Input: dimensioned drawing with shaded views. Units: mm. Origin: part minimum x, y, z. A direction names the side the tool comes from. Give positions to 0.01 mm unless a question says otherwise; leave off trailing zeros. Order: outer loops, then holes, each group sorted by start corner. A loop starts at its lowest first (then second) coordinate and runs counter-clockwise, first axis right, second up. Notation, with made-up numbers: M -14.5,26.5 L 28.5,26.5 A26 cw 28.5,49.5 Z; hole C 11.25,8.25 d6. An arc over 180 degrees is marked long. Answer in a Markdown table with one row per item. Add a question column.
(1) Pin query (flat end, axial travel): P1, Ø3.5, axis at x = 6.35, z = 6.35, coming from the +Y side. Return the tip coordinate at first contact, or that it passes through.
(2) Mould query, pull axis Z, two halves, no side actions, for the marked faces 1, 2 and 3. Classes: pulls with the +Z half, pulls with the -Z half, needs draft (parallel to the pull), parting line crosses it, or undercut.
(3) Material intervals for line 1 along X through (y, z) = (3.5, 6.35); line 2 along Y through (x, z) = (3.25, 2); line 3 along X through (y, z) = (8.75, 6.75) (1 decimal), sorted ascending.
(4) Section query B-B, the plane x = 7. Return loops of the section in (y, z).
(5) Set-up query: the marked faces 4 and 5. Return all of +Z, -Z, +X, -X, +Y, -Y with unobstructed straight access to the full face (end or side cutting, diameter ignored); none if empty.
(6) Section query A-A, the plane z = 6.35. Return loops of the section in (x, y).
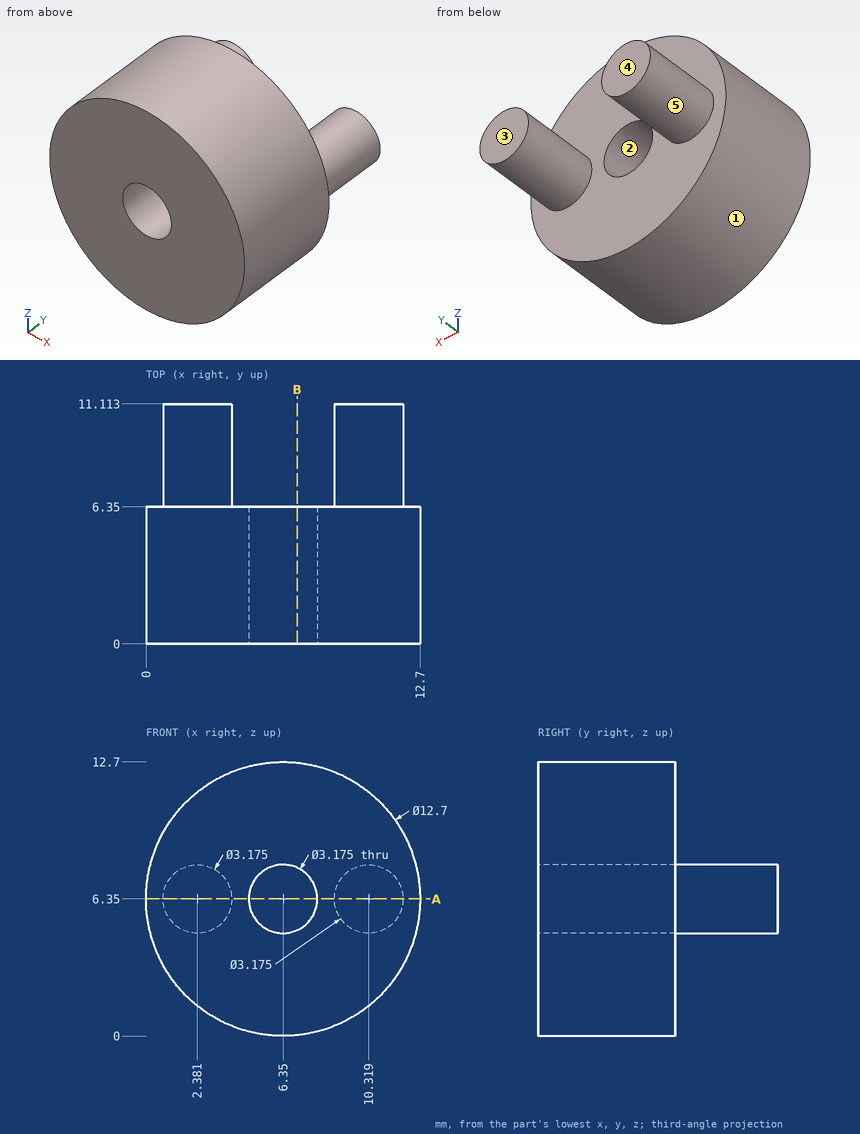
Values follow:
| question | item | result |
|---|---|---|
| 1 | P1 | stops at y = 6.35 |
| 2 | face 1 | parting line crosses it |
| 2 | face 2 | undercut |
| 2 | face 3 | needs draft |
| 3 | line 1 | x = 0 to 4.76, 7.94 to 12.7 |
| 3 | line 2 | y = 0 to 6.35 |
| 3 | line 3 | x = 0.8 to 3.9, 8.8 to 11.9 |
| 4 | outline | M 0,0.03 L 6.35,0.03 L 6.35,4.9 L 0,4.9 Z; M 0,7.8 L 6.35,7.8 L 6.35,12.67 L 0,12.67 Z |
| 5 | face 4 | +Z, -Z, +X, -X, +Y |
| 5 | face 5 | +Y |
| 6 | outline | M 0,0 L 4.76,0 L 4.76,6.35 L 3.97,6.35 L 3.97,11.11 L 0.79,11.11 L 0.79,6.35 L 0,6.35 Z; M 7.94,0 L 12.7,0 L 12.7,6.35 L 11.91,6.35 L 11.91,11.11 L 8.73,11.11 L 8.73,6.35 L 7.94,6.35 Z |
